The model under review builds one solid part; all positions refer to its coordinate system, in mm. Coordinates: 2 decimals unless noted, no trailing zeros. Write each loop counter-clockwise with the first axis right and the second up, starting at its lowest first coordinate (ties: lowest second). Pieces come first, ordered by that corner, then holes.
1) For line 1 (X direction, y = 0, z = 11.5); line 2 (Y direction, x = -3, z = 11.5); line 3 (Y direction, x = 0.75, z = 13), list the stretches that pass through material, from the lowest coordinate up.
2) Add section A-A, the plane z = 9.25. State the section outline as (x, y) points.
3) For P1, Ø2, axis at y = 2, z = 11.5, coming from the -X side; P2, Ø2, axis at x = 2, z = 8.5, coming from the -Y side; P3, Ø2, axis at x = 5, z = 6, coming from the +Y side, all flat-tipped, find the tip position at first contact; note any pin that passes through.
4) Add section B-B, the plane y = -0.25. Give the number of separate pieces and of enclosed holes in the cut face, then the cut area to 3 significant figures.
5) Mouldability with a two-part tool opening along Y and no side actions: class faces 1 (the cylindrical face through (3.6, -0.1, 9.1)), 2 (the cylindrical face through (-4.345, -0.208, 13.086)), 3 (the flat face through (-2, 2, 15)), 4 (the cylindrical face through (-7.583, -2.388, 8.922)) as released by +Y, released by -Y, zero draft, split by the parting line, or undercut.
from build123d import *

# Parameters (mm, degrees)
SKETCH051_R          = 7.95
SKETCH051_R_2        = 2.6
PAD016_DEPTH         = 12
SKETCH052_R          = 1.6
POCKET_DEPTH         = 8
CHAMFER_SIZE         = 0.4
BODY_PLACEMENT_ANGLE = 90


with BuildPart() as part:
    # Sketch051 → Pad016 (new body)
    with BuildSketch(Plane(origin=(0, 0, 0), x_dir=(0, 1, 0), z_dir=(0, 0, 1))):
        Circle(SKETCH051_R)
        with Locations((-1, 0)):
            Circle(SKETCH051_R_2, mode=Mode.SUBTRACT)
    extrude(amount=PAD016_DEPTH)

    # Sketch052 → Pocket (cut)
    with BuildSketch(Plane.XZ.offset(-8)):
        with Locations((0, 8.5)):
            Circle(SKETCH052_R)
    extrude(amount=POCKET_DEPTH, mode=Mode.SUBTRACT)

    # Chamfer
    chamfer_edges = [part.edges().sort_by_distance(p)[0] for p in [
        (0, -7.95, 0),
        (0, 7.95, 3.45),
        (1.131391, 7.869082, 7.368649),
        (1.131391, 7.869082, 9.631351),
        (0, 7.95, 11.05),
        (0, -7.95, 12),
        (-1.6, 7.787329, 8.5),
        (0, -3.6, 0),
    ]]
    chamfer(chamfer_edges, length=CHAMFER_SIZE)


with BuildPart() as part_1:
    # Body placement: moved
    add(part.part.moved(Location((0, 0, 3))).rotate(Axis((0, 0, 3), (0, 0, 1)), BODY_PLACEMENT_ANGLE))


solid = part_1.part
Geometry results:
1. line 1: x = 3.6 to 7.95
1. line 2: y = -7.36 to -1.6, 1.6 to 7.36
1. line 3: y = -7.91 to -2.59, 2.59 to 7.91
2. outline: circle Ø15.9 at (0, 0); hole circle Ø5.2 at (1, 0)
3. P1: stops at x = -7.76
3. P2: stops at y = -7.89
3. P3: stops at y = 6.87
4. separate pieces: 3
4. enclosed holes: 0
4. area: 108 mm2
5. face 1: undercut
5. face 2: undercut
5. face 3: zero draft
5. face 4: split by the parting line
